Study the drawing (mm; zero at the part's minimum x, y, z) and answer. A direction names the side the tool comes from. Give positions to 0.01 mm unless a question says otherwise; leave off trailing zeros. Write each loop counter-clockwise with the first axis right and the second up, starting at its lowest first coordinate (ties: lowest second). Pieces come first, ordered by that corner, then holes. Notation, with made-up numbers: M 10.25,30 L 51.25,30 A5 ccw 51.25,35 Z; hole C 45,83.5 d7. An arc over 180 degrees is marked long. Use a Markdown table: item, result. Add a question column.
Item 1: Given P1, Ø2, axis at y = 2.5, z = 5, coming from the -X side (1 decimal); P2, Ø3, axis at x = 5, y = 4.5, coming from the +Z side; P3, Ø1.5, axis at y = 3, z = 5, coming from the -X side, each flat-ended and moving along its own axis, determine where each tip first touches the part or whether it passes through.
Item 2: A cutting plane is placed at B-B on y = 0.65. Determine the outline of the cut face in (x, z).
Item 3: For the marked faces 5, 6 and 7, determine the directions among +Z, -Z, +X, -X, +Y, -Y from which every point of the face is accessible in a straight line to the end or side of a thin tool.
Item 4: Consider probe 1 along Z at (x, y) = (1, 1.3); probe 2 along Y at (x, z) = (2.75, 6.5); probe 3 along X at (y, z) = (3.6, 4.5). Determine where each line is inside the solid, lowest interval first. Write a range as [from, to].
Item 5: A cutting plane is placed at D-D on y = 2.7. Determine the outline of the cut face in (x, z).
Item 6: A cutting plane is placed at A-A on x = 2.25. Determine the outline of the cut face in (y, z), then the cut area to 3 significant figures.
Item 7: The mould has two halves that part along X. Classify the marked faces 1, 2, 3 and 4: pulls with the +X half, pulls with the -X half, needs draft (parallel to the pull), parting line crosses it, or undercut.
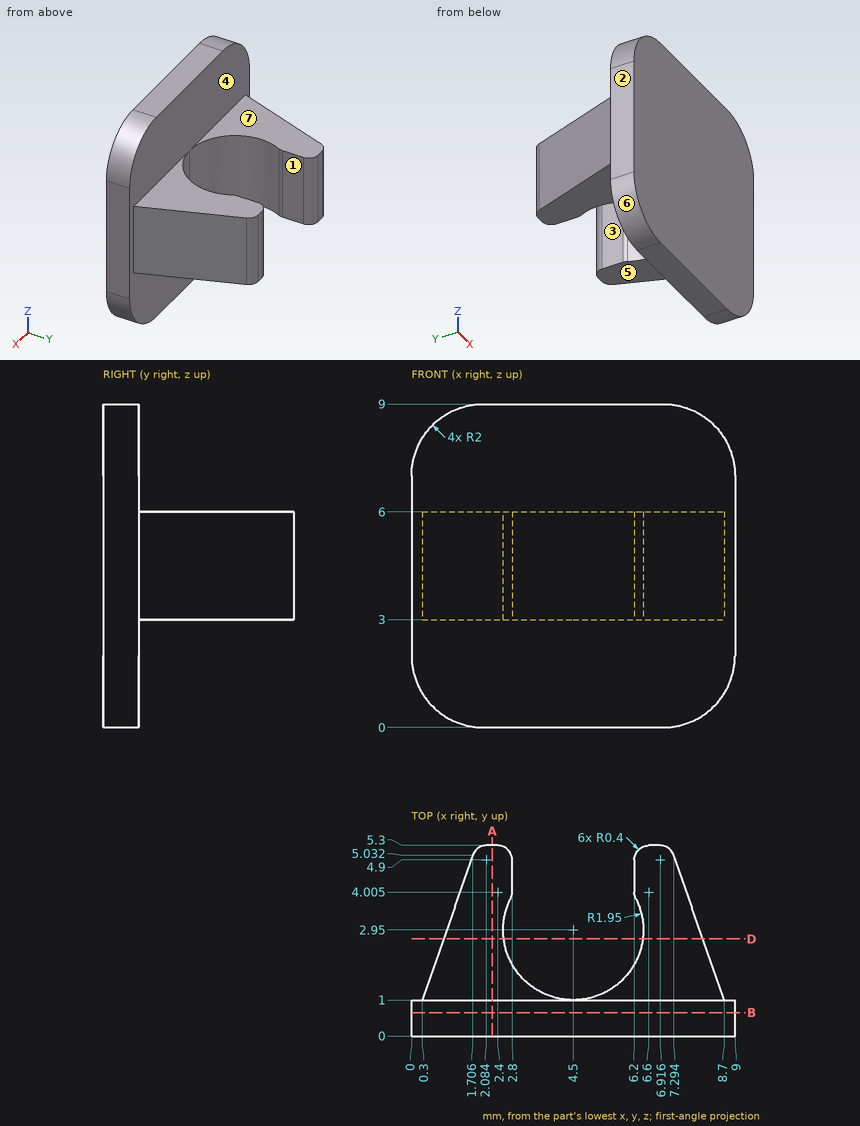
Filled in:
| question | item | result |
|---|---|---|
| 1 | P1 | x = 0.5 |
| 1 | P2 | z = 6 |
| 1 | P3 | x = 0.74 |
| 2 | outline | M 0,2 A2 ccw 2,0 L 7,0 A2 ccw 9,2 L 9,7 A2 ccw 7,9 L 2,9 A2 ccw 0,7 Z |
| 3 | face 5 | -Z, +X, -X, +Y |
| 3 | face 6 | -Z, -X, +Y, -Y |
| 3 | face 7 | +Z, +X, -X, +Y |
| 4 | probe 1 | [3, 6] |
| 4 | probe 2 | [0, 1] |
| 4 | probe 3 | [1.21, 2.66], [6.34, 7.79] |
| 5 | outline | M 0.89,3 L 2.57,3 L 2.57,6 L 0.89,6 Z; M 6.43,3 L 8.11,3 L 8.11,6 L 6.43,6 Z |
| 6 | outline | M 0,0 L 1,0 L 1,3 L 5.3,3 L 5.3,6 L 1,6 L 1,9 L 0,9 Z |
| 6 | area | 21.9 mm² |
| 7 | face 1 | undercut |
| 7 | face 2 | pulls with the -X half |
| 7 | face 3 | undercut |
| 7 | face 4 | needs draft |
